Read the model definition and answer for the solid it produces. Units are mm, in the model's axes. A direction names the side the tool comes from. Coordinates: 2 decimals unless noted, no trailing zeros. Order: outer loops, then holes, each group sorted by start corner. A loop starts at its lowest first (then second) coordinate and runs counter-clockwise, first axis right, second up.
```python
from build123d import *

# Parameters (mm, degrees)
BOSS_EXTRUDE1_DEPTH      = 25
BOSS_EXTRUDE1_DEPTH_BACK = 10
SKETCH1_R                = 10
SKETCH2_R                = 12.5
BOSS_EXTRUDE2_DEPTH      = 25
BOSS_EXTRUDE3_DEPTH      = 15
BOSS_EXTRUDE3_DEPTH_BACK = 15
CUT_EXTRUDE1_DEPTH       = 10
SKETCH7_R                = 10.5
BOSS_EXTRUDE4_DEPTH      = 3.175
CUT_EXTRUDE2_DEPTH       = 10
SKETCH11_R               = 5
CUT_EXTRUDE6_DEPTH       = 10


with BuildPart() as part:
    # Sketch1 → Boss-Extrude1 (new, two sides: drawn at the far end of the back side and taken through both)
    with BuildSketch(Plane(origin=(0, 0, 0), x_dir=(0, 0, -1), z_dir=(1, 0, 0)).offset(-BOSS_EXTRUDE1_DEPTH_BACK)):
        Circle(SKETCH1_R)
    extrude(amount=BOSS_EXTRUDE1_DEPTH + BOSS_EXTRUDE1_DEPTH_BACK)

    # Sketch2 → Boss-Extrude2 (add, symmetric)
    with BuildSketch(Plane(origin=(-10, 0, 0), x_dir=(0.9848069802426886, -0.173652560203633, 1.5808464272800858e-08), z_dir=(0.17364817766692736, 0.9847821256419462, -0.007104604780387524))):
        with Locations(Location((0, 0, 0), (0, 0, 180.000000906))):
            Circle(SKETCH2_R)
    extrude(amount=BOSS_EXTRUDE2_DEPTH, both=True)

    # Sketch5 → Boss-Extrude3 (add, two sides: drawn at the far end of the back side and taken through both)
    with BuildSketch(Plane(origin=(0, 0, 0), x_dir=(0, 0, -1), z_dir=(1, 0, 0)).offset(-BOSS_EXTRUDE3_DEPTH_BACK)):
        Polygon((0.79375, -1.374815329), (-0.79375, 1.374815329), (-25.529710951, -12.906498385), (-23.942210951, -15.656129042), align=None)
    extrude(amount=BOSS_EXTRUDE3_DEPTH + BOSS_EXTRUDE3_DEPTH_BACK)

    # Sketch6 → Cut-Extrude1 (cut)
    with BuildSketch(Plane(origin=(0, -1.374815329, -0.79375), x_dir=(1, 0, 0), z_dir=(0, -0.8660254037844415, -0.4999999999999954))):
        Polygon((15, 28.562627427), (15, 10), (8.243756147, 28.562627427), align=None)
    extrude(amount=-CUT_EXTRUDE1_DEPTH, mode=Mode.SUBTRACT)

    # Sketch7 → Boss-Extrude4 (add)
    with BuildSketch(Plane.XZ.offset(15.656129042)):
        with BuildLine():
            Line((-14.420950658, 73.942210951), (-15, 23.942210951))
            Line((-15, 23.942210951), (8.243756147, 23.942210951))
            ThreePointArc((8.243756147, 23.942210951), (7.001386396, 27.211000098), (6.579049342, 30.68232499))
            Line((6.579049342, 30.68232499), (6.579049342, 73.942210951))
            ThreePointArc((6.579049342, 73.942210951), (-3.920950658, 63.442210951), (-14.420950658, 73.942210951))
        make_face()
        with Locations((-3.920950658, 73.942210951)):
            Circle(SKETCH7_R)
    extrude(amount=-BOSS_EXTRUDE4_DEPTH)

    # Sketch9 → Cut-Extrude2 (cut)
    with BuildSketch(Plane.XZ.offset(15.656129042)):
        with BuildLine():
            Line((17.296769939, 44.662823633), (24.815608182, 16.701826347))
            ThreePointArc((24.815608182, 16.701826347), (7.075690418, 26.922905868), (17.296769939, 44.662823633))
        make_face()
    extrude(amount=-CUT_EXTRUDE2_DEPTH, mode=Mode.SUBTRACT)

    # Sketch11 → Cut-Extrude6 (cut)
    with BuildSketch(Plane(origin=(0, -12.481129042, 0), x_dir=(1, 0, 0), z_dir=(0, 1, 0))):
        with Locations(Location((-3.920950658, -73.942210951, 0), (0, 0, 270))):
            Circle(SKETCH11_R)
    extrude(amount=-CUT_EXTRUDE6_DEPTH, mode=Mode.SUBTRACT)


solid = part.part
```
1) A cutting plane is placed at B-B, the plane z = 17. Determine the outline of the cut face in (x, y), and give its area (3 significant figures).
A:
outline: (-15, -11.65) - (11.16, -11.65) - (11.83, -7.98) - (-15, -7.98) - close
area: 97.1 mm2
2) Straight lines are drawn through the part: line 1 (Y direction, x = -10, z = 60.5); line 2 (Z direction, x = -2.5, y = -8); line 3 (Z direction, x = 16, y = 0.5). For each, find the intervals that lie inside material, in ascending order.
A:
line 1: y = -15.66 to -12.48
line 2: z = -8.86 to 8.95, 10.68 to 17.03
line 3: z = -9.99 to 9.99
3) Flat-ended cylindrical pins translate along their axes: pin 1 Ø7 at (x, z) = (-2.5, 61.5) entering from +Y; pin 2 Ø13 at (x, z) = (-3.92, 73.94) entering from -Y; pin 3 Ø6 at (x, z) = (11, 60) entering from -Y (3 decimals); pin 4 Ø2.5 at (y, z) = (-14, 52) entering from +X. Find the tip coordinate at first contact, or state that the pin passes through.
A:
pin 1: stops at y = -12.48
pin 2: stops at y = -15.66
pin 3: passes through
pin 4: stops at x = 6.58
4) Determine the mould class of faces 1 (the flat face through (-4, -15.656, 55)), 2 (the cylindrical face through (-3.69, -14.09, 84.44)), 3 (the cylindrical face through (-3.701, -14.046, 68.947)) for opening direction Z: pulls with the +Z half, pulls with the -Z half, needs draft (parallel to the pull), parting line crosses it, or undercut.
A:
face 1: needs draft
face 2: pulls with the +Z half
face 3: undercut
5) A cutting plane is placed at A-A, the plane z = 67.5. Determine the outline of the cut face in (x, y).
A:
outline: (-14.5, -15.66) - (6.58, -15.66) - (6.58, -12.48) - (-14.5, -12.48) - close
6) Which of the six approach directions +Z, -Z, +X, -X, +Y, -Y give full straight-line access (tool end or side, diameter ignored) to faces 4 (the flat face through (-4, -12.481, 55)), 5 (the cylindrical face through (14.11, 3, -9.54)), 6 (the flat face through (12.42, -8.56, 14.79)), 7 (the flat face through (25, 0, 0)), 8 (the flat face through (6.579, -14, 52))?
A:
face 4: +Z, +X, -X, +Y
face 5: +X
face 6: +Z, +X, -Y
face 7: +Z, -Z, +X, +Y, -Y
face 8: +Z, +X, +Y, -Y
